Part print with two shaded views. Sizes in mm from the minimum x, y, z corner. Round coordinates to 2 decimals unless told otherwise and drop trailing zeros. Return JSON: item names as keys, results as strings. Group by question number.
Item 1: Pull direction X, two halves, no side cores. Call the marked faces 1, 2 and 3: pulls with the +X half, pulls with the -X half, needs draft (parallel to the pull), parting line crosses it, or undercut.
Item 2: Probe line 1 along X through (y, z) = (4, 17.5) (1 decimal); line 2 along X through (y, z) = (1.5, 15.5) (1 decimal); line 3 along Z through (x, y) = (48, 3). List the from-to ranges inside material, lowest first.
Item 3: Pin check, flat tip, straight feed: pin 1 Ø3 at (x, z) = (49.21, 15.88) entering from -Y. Stop position of the tip, or through.
Item 4: Slice it at A-A on y = 3.5. Give the number of separate pieces and of enclosed holes in the cut face, then the cut area to 3 significant figures.
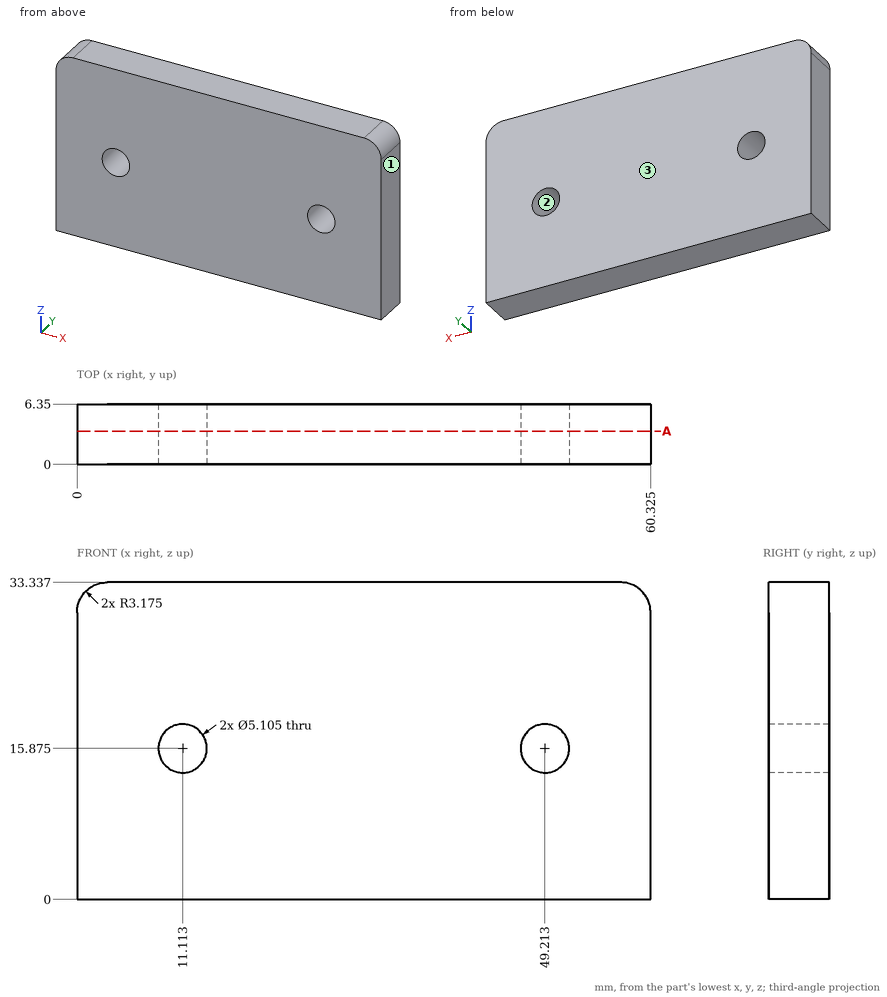
Output values:
{
 "1": {"face 1": "pulls with the +X half", "face 2": "undercut", "face 3": "needs draft"},
 "2": {"line 1": "0 to 9.1, 13.1 to 47.2, 51.2 to 60.3", "line 2": "0 to 8.6, 13.6 to 46.7, 51.7 to 60.3", "line 3": "0 to 13.63, 18.12 to 33.34"},
 "3": {"pin 1": "through"},
 "4": {"separate pieces": "1", "enclosed holes": "2", "area": "1,970 mm²"}
}
